Geometry: see drawing. Coordinates: mm, zero at the bounding-box minimum. Coordinates: 2 decimals unless noted, no trailing zeros. Write each loop counter-clockwise with the first axis right and the second up, starting at its lowest first coordinate (ties: lowest second). Pieces come first, ordered by that corner, then holes. Notation, with made-up numbers: M -11.75,76.25 L 8.25,76.25 A9 ccw 8.25,93.25 Z; hole C 84.25,56.25 d11. An arc over 180 degrees is marked long. Answer as CSV lines item,"result". Start each with the question number.
1. Contact query for flat-ended pins moving along their axis: pin 1 Ø2.5 at (x, z) = (78, 11) entering from -Y; pin 2 Ø1 at (x, z) = (83.5, 15.5) entering from +Y. Output: stop coordinate, or through.
2. Line query: probe 1 along Z at (x, y) = (47.5, 14.75); probe 2 along Y at (x, z) = (47.5, 4.25); probe 3 along Y at (x, z) = (51.5, 14.5). Output: solid intervals per line, ascending. Write a range as [from, to].
3. Mould query, pull axis X, two halves, no side actions, for the marked faces 1, 2 and 3. Classes: pulls with the +X half, pulls with the -X half, needs draft (parallel to the pull), parting line crosses it, or undercut.
4. Section C-C on y = 9. Return the cut outline in (x, z).
5. Section B-B on x = 47.5. Return the cut outline in (y, z).
6. Section A-A on y = 40. Return the cut outline in (x, z), plus the area to 3 significant figures.
7. Section D-D on x = 62. Return the cut outline in (y, z), plus the area to 3 significant figures.
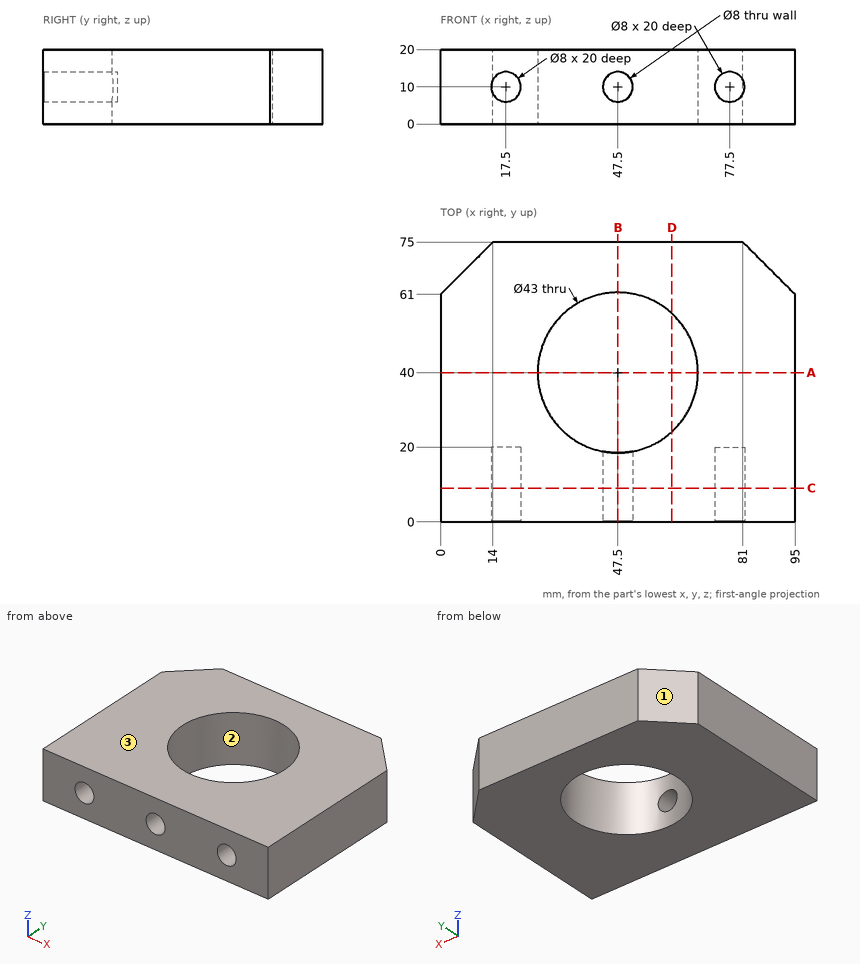
Values:
1,pin 1,"y = 20"
1,pin 2,"y = 73"
2,probe 1,"[0, 6], [14, 20]"
2,probe 2,"[0, 18.5], [61.5, 75]"
2,probe 3,"[0, 18.88], [61.12, 75]"
3,face 1,"pulls with the -X half"
3,face 2,"undercut"
3,face 3,"needs draft"
4,outline,"M 0,0 L 95,0 L 95,20 L 0,20 Z; hole C 17.5,10 d8; hole C 47.5,10 d8; hole C 77.5,10 d8"
5,outline,"M 0,0 L 18.5,0 L 18.5,6 L 0,6 Z; M 0,14 L 18.5,14 L 18.5,20 L 0,20 Z; M 61.5,0 L 75,0 L 75,20 L 61.5,20 Z"
6,outline,"M 0,0 L 26,0 L 26,20 L 0,20 Z; M 69,0 L 95,0 L 95,20 L 69,20 Z"
6,area,"1,040 mm²"
7,outline,"M 0,0 L 24.13,0 L 24.13,20 L 0,20 Z; M 55.87,0 L 75,0 L 75,20 L 55.87,20 Z"
7,area,"865 mm²"
